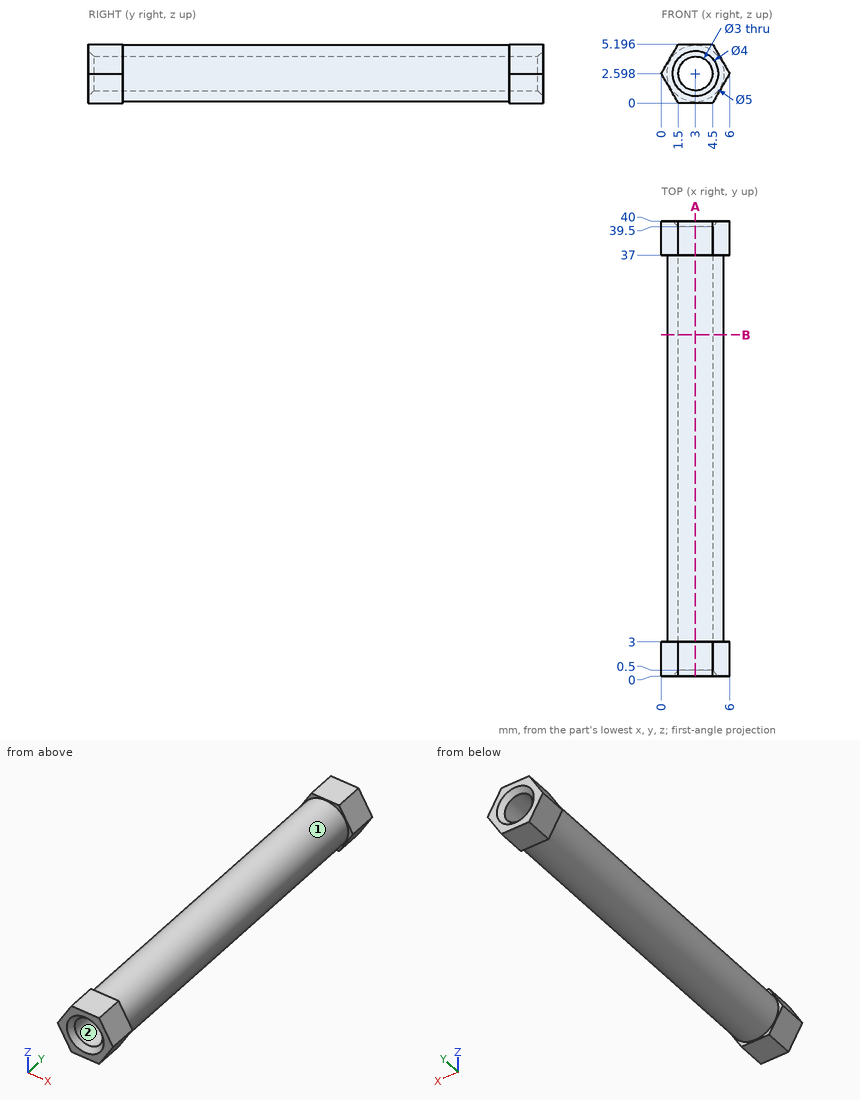
The drawing under review shows one solid part. Ordinate dimensions are in mm from its lowest x, y, z. Coordinates: 2 decimals unless noted, no trailing zeros. Write each loop counter-clockwise with the first axis right and the second up, starting at its lowest first coordinate (ties: lowest second). Pieces come first, ordered by that corner, then holes. Notation, with made-up numbers: M 6.25,77 L 42.25,77 A10 ccw 42.25,96 Z; hole C -21,-29.75 d3. An arc over 180 degrees is marked long. Answer as a JSON object with one key per item and string values.
Item 1: Draft analysis for pull direction Y (two halves, no side actions). For the marked faces 1 and 2, state which applies: pulls with the +Y half, pulls with the -Y half, needs draft (parallel to the pull), parting line crosses it, or undercut.
Outcome:
{"face 1": "undercut", "face 2": "needs draft"}
Item 2: Wall thickness on probe 1 along Z at (x, y) = (3, 21); probe 2 along Y at (x, z) = (4.8, 0.8); probe 3 along X at (y, z) = (33.5, 1.7): over which ranges is each line inside the solid? List them lowest first.
Outcome:
{"probe 1": "0.1 to 1.1, 4.1 to 5.1", "probe 2": "0 to 3, 37 to 40", "probe 3": "0.67 to 1.8, 4.2 to 5.33"}
Item 3: Add section A-A, the plane x = 3. Give the boundary of the cut face in (y, z).
Outcome:
{"outline": "M 0,0 L 3,0 L 3,0.1 L 37,0.1 L 37,0 L 40,0 L 40,0.6 L 39.5,1.1 L 0.5,1.1 L 0,0.6 Z; M 0,4.6 L 0.5,4.1 L 39.5,4.1 L 40,4.6 L 40,5.2 L 37,5.2 L 37,5.1 L 3,5.1 L 3,5.2 L 0,5.2 Z"}
Item 4: Add section B-B, the plane y = 30. Give the boundary of the cut face in (x, z).
Outcome:
{"outline": "C 3,2.6 d5; hole C 3,2.6 d3"}
Item 5: Insertion check: pin 1 Ø1 at (y, z) = (26.5, 1) entering from -X; pin 2 Ø3 at (x, y) = (2.5, 9) entering from +Z. Each pin has a flat end and moves straight along its axis. Give the tip position at first contact, or say it passes through.
Outcome:
{"pin 1": "x = 0.75", "pin 2": "z = 5.1"}
